from build123d import *

# Parameters (mm, degrees)
SKETCH_W        = 20.1
SKETCH_H        = 8.5
SKETCH_R        = 1.3
PAD_DEPTH       = 6
POCKET_DEPTH    = 3
PAD001_DEPTH    = 9
SKETCH003_R     = 1.6
POCKET001_DEPTH = 5
POCKET002_DEPTH = 3.8
SKETCH005_R     = 2.7
POCKET003_DEPTH = 3


with BuildPart() as pocket003:
    # Sketch → Pad (new body)
    with BuildSketch(Plane.XY):
        with Locations((10.05, 4.25)):
            Rectangle(SKETCH_W, SKETCH_H)
        with Locations((7.2, 4.25)):
            Circle(SKETCH_R, mode=Mode.SUBTRACT)
    extrude(amount=PAD_DEPTH)

    # Sketch001 → Pocket (cut)
    with BuildSketch(Plane(origin=(0, 0, 0), x_dir=(1, 0, 0), z_dir=(0, 0, -1))):
        Polygon((5.721983, -1.69), (8.678017, -1.69), (10.156033, -4.25), (8.678017, -6.81), (5.721983, -6.81), (4.243967, -4.25), align=None)
    extrude(amount=-POCKET_DEPTH, mode=Mode.SUBTRACT)

    # Sketch002 → Pad001 (new body)
    with BuildSketch(Plane(origin=(0, 0, 0), x_dir=(0, -1, 0), z_dir=(-1, 0, 0))):
        with BuildLine():
            ThreePointArc((1.92947, -6.231983), (-4.5, -2), (-10.92947, -6.231983))
            Line((-10.92947, -6.231983), (-22.64647, -6.231983))
            Line((-22.64647, -1.231983), (-22.64647, -6.231983))
            Line((-13.64647, -1.231983), (-22.64647, -1.231983))
            ThreePointArc((4.64647, -1.231983), (-4.5, 3), (-13.64647, -1.231983))
            Line((13.64647, -1.231983), (4.64647, -1.231983))
            Line((13.64647, -6.231983), (13.64647, -1.231983))
            Line((13.64647, -6.231983), (1.92947, -6.231983))
        make_face()
    extrude(amount=PAD001_DEPTH)

    # Sketch003 → Pocket001 (cut)
    with BuildSketch(Plane.XY.offset(-1.231983)):
        with Locations((-4.5, 18.14647)):
            Circle(SKETCH003_R)
        with Locations((-4.5, -9.14647)):
            Circle(SKETCH003_R)
    extrude(amount=-POCKET001_DEPTH, mode=Mode.SUBTRACT)

    # Sketch004 → Pocket002 (cut)
    with BuildSketch(Plane.XY.offset(-1.231983)):
        Polygon((-6.116581, -6.34647), (-2.883419, -6.34647), (-1.266838, -9.14647), (-2.883419, -11.94647), (-6.116581, -11.94647), (-7.733162, -9.14647), align=None)
    extrude(amount=-POCKET002_DEPTH, mode=Mode.SUBTRACT)

    # Sketch005 → Pocket003 (cut)
    with BuildSketch(Plane.XY.offset(-1.231983)):
        with Locations((-4.5, 18.14647)):
            Circle(SKETCH005_R)
    extrude(amount=-POCKET003_DEPTH, mode=Mode.SUBTRACT)


with BuildPart() as part_mirroring:
    # Part__Mirroring: instance of Pocket003
    add(pocket003.part.mirror(Plane(origin=(0, 0, 0), x_dir=(0, -1, 0), z_dir=(1, 0, 0))))


with BuildPart() as part_mirroring_1:
    # Part__Mirroring placement: moved
    add(part_mirroring.part.moved(Location((40.1, 0, 0))))


with BuildPart() as fusion:
    # Fusion base: copy of Pocket003
    add(pocket003.part)

    # Fusion: union Part__Mirroring
    add(part_mirroring_1.part)


solid = fusion.part
Design review of the part built by this model. Coordinates are the model's own, in mm. A direction names the side the tool comes from. Round coordinates to 2 decimals unless told otherwise and drop trailing zeros. Order: outer loops, then holes, each group sorted by start corner. A loop starts at its lowest first (then second) coordinate and runs counter-clockwise, first axis right, second up.
1) Consider section D-D (y = 13). State the section outline as (x, z) points, plus the area to 3 significant figures.
The answers:
outline: (-9, -6.23) - (0, -6.23) - (0, -0.53) - (-9, -0.53) - close; (40.1, -6.23) - (49.1, -6.23) - (49.1, -0.53) - (40.1, -0.53) - close
area: 103 mm2
2) Consider section C-C (z = 4). State the section outline as (x, y) points.
The answers:
outline: (0, 0) - (40.1, 0) - (40.1, 8.5) - (0, 8.5) - close; hole circle Ø2.6 at (7.2, 4.25); hole circle Ø2.6 at (32.9, 4.25)
3) Clearance check with flat-ended pins moving along their axes: pin 1 Ø10 at (x, y) = (23.5, -8) entering from +Z; pin 2 Ø1.5 at (x, z) = (33, 1) entering from +Y; pin 3 Ø5 at (x, y) = (1, -10) entering from +Z; pin 4 Ø1.2 at (y, z) = (5.5, 4) entering from +X. State where each tip first meets the part, or that it passes through.
The answers:
pin 1: passes through
pin 2: stops at y = 8.5
pin 3: stops at z = -1.23
pin 4: stops at x = 40.1
4) Consider section A-A (x = 44.6). State the section outline as (y, z) points, plus the area to 3 significant figures.
The answers:
outline: (-13.65, -6.23) - (-10.75, -6.23) - (-10.75, -5.03) - (-11.95, -5.03) - (-11.95, -1.23) - (-13.65, -1.23) - close; (-7.55, -6.23) - (-1.93, -6.23) arc R7 cw to (10.93, -6.23) - (16.55, -6.23) - (16.55, -4.23) - (15.45, -4.23) - (15.45, -1.23) - (13.65, -1.23) arc R12 ccw to (-4.65, -1.23) - (-6.35, -1.23) - (-6.35, -5.03) - (-7.55, -5.03) - close; (19.75, -6.23) - (22.65, -6.23) - (22.65, -1.23) - (20.85, -1.23) - (20.85, -4.23) - (19.75, -4.23) - close
area: 148 mm2
5) Consider section B-B (x = 7.2). State the section outline as (y, z) points, plus the area to 3 significant figures.
The answers:
outline: (0, 0) - (1.69, 0) - (1.69, 3) - (2.95, 3) - (2.95, 6) - (0, 6) - close; (5.55, 3) - (6.81, 3) - (6.81, 0) - (8.5, 0) - (8.5, 6) - (5.55, 6) - close
area: 27.8 mm2
6) Draft analysis for pull direction Y (two halves, no side actions). For faces 1 (the flat face through (43.5, 16.7, -6.232)), 2 (the flat face through (45, 22.646, -4)), 3 (the flat face through (46, -8, -5.032)), state which applies: released by +Y, released by -Y, zero draft, split by the parting line, or undercut.
The answers:
face 1: zero draft
face 2: released by +Y
face 3: undercut
7) For L1, parallel to X at y = 4.25, z = 5.4; L2, parallel to X at y = 14, z = -4.5; L3, parallel to Y at x = 32.9, z = 4.4, list the stretches that pass through material, from the lowest coordinate up.
The answers:
L1: x = 0 to 5.9, 8.5 to 31.6, 34.2 to 40.1
L2: x = -9 to 0, 40.1 to 49.1
L3: y = 0 to 2.95, 5.55 to 8.5
8) Machinability: for faces 4 (the flat face through (9.407, 2.952, 1.479)), 5 (the flat face through (45, -7, -6.232)), 6 (the flat face through (45, -6.346, -3)), 7 (the flat face through (-2, 20, -1.232)), 8 (the flat face through (44.5, -12.2, -1.232)), which of the approach directions +Z, -Z, +X, -X, +Y, -Y give a long, thin tool a straight path to every point of the face, cutting with its end or side? Answer none if there is none.
The answers:
face 4: -Z
face 5: -Z, +X, -X, +Y, -Y
face 6: +Z
face 7: +Z, +X, -X, +Y
face 8: +Z, +X, -X, -Y
